Geometry: final body of the model. Coordinates: model frame, mm. A direction names the side the tool comes from. Give positions to 0.01 mm unless a question says otherwise; leave off trailing zeros. Write each loop counter-clockwise with the first axis right and the second up, starting at its lowest first coordinate (ties: lowest second). Pieces come first, ordered by that corner, then holes. Notation, with made-up numbers: (69, 79) - (75, 79) arc R10 cw to (75, 92) - close; hole circle Ø7 at (-36, 42). An arc over 180 degrees is marked (long way). Use CSV: the item, a comma, the result in double quotes. Start each with the question number.
(1) Reachability of faces 4 (the flat face through (-72, 46.125, 3)), 5 (the flat face through (-46.125, -72, 3)), 6 (the flat face through (15.375, -72, 3)) from +Z, -Z, +X, -X, +Y, -Y: full face, straight path, thin tool, end or side. Return the list, or none.
(2) Section A-A on y = 0. Output: boundary loops of the cut face in (x, z), and give its area (3 significant figures).
(3) Section C-C on x = 11.5. Output: boundary loops of the cut face in (y, z), and give its area (3 significant figures).
(4) Draft query along Y for faces 1 (the flat face through (15.375, 72, 3)), 2 (the flat face through (-72, -46.125, 3)), 3 (the flat face through (72, 15.375, 3)). Return one class per face: released by +Y, released by -Y, zero draft, split by the parting line, or undercut.
(5) Line query: probe 1 along Y at (x, z) = (-28, 1.45); probe 2 along X at (y, z) = (-9, 4); probe 3 along Y at (x, z) = (54, 2.65). Output: solid intervals per line, ascending. Write a range as [from, to].
(6) Section B-B on x = -28. Output: boundary loops of the cut face in (y, z), and give its area (3 significant figures).
(7) Section D-D on z = 0.95. Count the separate pieces of the cut face and the enclosed holes in it, and give its area (3 significant figures).
(8) First-contact query: pin 1 Ø3 at (y, z) = (-0.5, 1.5) entering from +X; pin 2 Ø1 at (x, z) = (-1, 1.5) entering from -Y. Flat tips, straight axial feed; report the tip coordinate or a pass-through.
Autodesk Inventor part; units mm, degrees
ref_plane "YZ Plane" through (0, 0, 0) normal (1, 0, 0) x (0, 1, 0)
ref_plane "XZ Plane" through (0, 0, 0) normal (0, 1, 0) x (-1, 0, 0)
ref_plane "XY Plane" through (0, 0, 0) normal (0, 0, 1) x (1, 0, 0)
sketch "Sketch1" plane through (0, 0, 0) normal (0, 0, 1) x (1, 0, 0)
  line L0 (-75, -15.375) -> (-69, -15.375)
  line L1 (-69, -46.125) -> (-75, -46.125)
  line L2 (-69, 46.125) -> (-75, 46.125)
  line L3 (-75, 15.375) -> (-69, 15.375)
  line L4 (-69, 46.125) -> (-69, 69)
  line L5 (-75, 46.125) -> (-75, 15.375)
  line L6 (-69, 15.375) -> (-69, -15.375)
  line L7 (-75, -15.375) -> (-75, -46.125)
  line L8 (-69, -46.125) -> (-69, -69)
  line L9 (0, 0) -> (0, 15.375)
  line L10 (0, 0) -> (0, -46.125)
  line L11 (69, 15.375) -> (69, -15.375)
  line L12 (75, 15.375) -> (69, 15.375)
  line L13 (75, 46.125) -> (75, 15.375)
  line L14 (69, 46.125) -> (75, 46.125)
  line L15 (69, 46.125) -> (69, 69)
  line L16 (75, -15.375) -> (69, -15.375)
  line L17 (75, -15.375) -> (75, -46.125)
  line L18 (69, -46.125) -> (75, -46.125)
  line L19 (69, -46.125) -> (69, -69)
  line L20 (0, 0) -> (92.4518, 92.4518)
  line L21 (0, 0) -> (130.7466, 0) construction
  line L22 (0, 0) -> (109.2471, 0) construction
  line L23 (0, 0) -> (102.0745, -102.0745)
  line L24 (0, 0) -> (162.0274, 0) construction
  line L25 (15.375, 69) -> (-15.375, 69)
  line L26 (15.375, 75) -> (15.375, 69)
  line L27 (46.125, 75) -> (15.375, 75)
  line L28 (46.125, 69) -> (46.125, 75)
  line L29 (46.125, 69) -> (69, 69)
  line L30 (-15.375, 75) -> (-15.375, 69)
  line L31 (-15.375, 75) -> (-46.125, 75)
  line L32 (-46.125, 69) -> (-46.125, 75)
  line L33 (-46.125, 69) -> (-69, 69)
  line L34 (-15.375, -75) -> (-15.375, -69)
  line L35 (-46.125, -69) -> (-46.125, -75)
  line L36 (46.125, -69) -> (46.125, -75)
  line L37 (15.375, -75) -> (15.375, -69)
  line L38 (46.125, -69) -> (69, -69)
  line L39 (46.125, -75) -> (15.375, -75)
  line L40 (15.375, -69) -> (-15.375, -69)
  line L41 (-15.375, -75) -> (-46.125, -75)
  line L42 (-46.125, -69) -> (-69, -69)
  line L43 (0, 0) -> (-28, 0)
  circle A0 centre (-28, 0) radius 20
  line L44 (0, 0) -> (45, 0)
  line L45 (35, 10) -> (55, 10)
  line L46 (55, 10) -> (55, -10)
  line L47 (55, -10) -> (35, -10)
  line L48 (35, -10) -> (35, 10)
  line L49 (35, 10) -> (55, -10) construction
  line L50 (55, 10) -> (35, -10) construction
  point P0 (0, 0)
  point P1 (-69, -75)
  point P2 (-69, 75)
  point P3 (69, -75)
  point P4 (69, 75)
  dimension "d8" = 45
  dimension "d13" = 28
  dimension "d14" = 40
  dimension "d15" = 45
  dimension "d16" = 20
  dimension "d17" = 20
extrude "Extrusion1" add sketch "Sketch1" along normal blind 6
properties part number "Bottom"
Check values:
1,face 4,"+Z, -Z, -X, +Y"
1,face 5,"+Z, -Z, -X, -Y"
1,face 6,"+Z, -Z, -Y"
2,outline,"(-69, 0) - (-48, 0) - (-48, 6) - (-69, 6) - close; (-8, 0) - (35, 0) - (35, 6) - (-8, 6) - close; (55, 0) - (69, 0) - (69, 6) - (55, 6) - close"
2,area,"468 mm²"
3,outline,"(-69, 0) - (69, 0) - (69, 6) - (-69, 6) - close"
3,area,"828 mm²"
4,face 1,"zero draft"
4,face 2,"released by -Y"
4,face 3,"undercut"
5,probe 1,"y = [-75, -20], [20, 75]"
5,probe 2,"x = [-69, -45.86], [-10.14, 35], [55, 69]"
5,probe 3,"y = [-69, -10], [10, 69]"
6,outline,"(-75, 0) - (-20, 0) - (-20, 6) - (-75, 6) - close; (20, 0) - (75, 0) - (75, 6) - (20, 6) - close"
6,area,"660 mm²"
7,separate pieces,"1"
7,enclosed holes,"2"
7,area,"18,900 mm²"
8,pin 1,"stops at x = 69"
8,pin 2,"stops at y = -69"
